Part model, mm, in its own coordinate system. A direction names the side the tool comes from. Coordinates: 2 decimals unless noted, no trailing zeros. Write each loop counter-clockwise with the first axis right and the second up, starting at its lowest first coordinate (ties: lowest second). Pieces come first, ordered by that corner, then holes. Notation, with made-up numbers: (49, 64) - (63, 64) arc R26 ccw to (63, 90) - close; hole circle Ø9 at (43, 56). An arc over 180 degrees is marked (long way). Use a Markdown table: item, result.
Autodesk Inventor part; units mm, degrees
ref_plane "Work Plane2" through (-20, 0, -10) normal (0, 0, 1) x (1, 0, 0)
ref_plane "Work Plane3" through (0, 8, 0) normal (0, 1, 0) x (1, 0, 0)
ref_plane "YZ Plane" through (0, 0, 0) normal (1, 0, 0) x (0, 1, 0)
sketch "Sketch1" plane through (0, 0, 0) normal (0, 1, 0) x (-1, 0, 0)
  line L0 (0, 0) -> (20, 0)
  line L1 (20, 0) -> (20, -20)
  line L2 (20, -20) -> (0, -20)
  line L3 (0, -20) -> (0, 0)
  dimension "d0" = 20
  dimension "d1" = 20
extrude "Extrusion1" add sketch "Sketch1" along normal blind 10
sketch "Sketch4" plane through (0, 10, 0) normal (0, 1, 0) x (1, 0, 0)
  line L0 (0, 20) -> (-20, 20)
  line L1 (-20, 20) -> (-20, 0)
  line L2 (-20, 0) -> (0, 0)
  line L3 (0, 0) -> (0, 20)
  line L4 (0, 20) -> (-20, 20)
  line L5 (-20, 20) -> (0, 0)
  line L6 (-10.1768, 10.1768) -> (-7.7019, 12.6517)
  line L7 (-7.7019, 12.6517) -> (-5.227, 10.1768)
  line L8 (-5.227, 10.1768) -> (-7.7019, 7.7019)
  line L9 (-7.7019, 7.7019) -> (-10.1768, 10.1768)
  line L10 (-10.1768, 10.1768) -> (-12.6517, 7.7019)
  line L11 (-12.6517, 7.7019) -> (-15.1265, 10.1768)
  line L12 (-15.1265, 10.1768) -> (-12.6517, 12.6517)
  line L13 (-12.6517, 12.6517) -> (-10.1768, 10.1768)
  line L14 (-12.6517, 12.6517) -> (-10.1768, 15.1265)
  line L15 (-10.1768, 15.1265) -> (-7.7019, 12.6517)
  line L16 (-7.7019, 12.6517) -> (-10.1768, 10.1768)
  line L17 (-10.1768, 10.1768) -> (-12.6517, 12.6517)
  line L18 (-12.6517, 7.7019) -> (-10.1768, 10.1768)
  line L19 (-10.1768, 10.1768) -> (-7.7019, 7.7019)
  line L20 (-7.7019, 7.7019) -> (-10.1768, 5.227)
  line L21 (-10.1768, 5.227) -> (-12.6517, 7.7019)
  dimension "d10" = 3.5
  dimension "d11" = 3.5
  dimension "d12" = 3.5
  dimension "d13" = 3.5
extrude "Extrusion3" cut sketch "Sketch4" against normal blind 8 contours L14 L15 L6 L5 | L5 L10 L11 L12 | L20 L21 L10 L5 | L5 L6 L7 L8
sketch "Sketch5" plane through (0, 10, 0) normal (0, 1, 0) x (1, 0, 0)
  line L0 (-5.227, 10.1768) -> (-10.1768, 5.227)
  line L1 (-10.1768, 5.227) -> (-15.1265, 10.1768)
  line L2 (-15.1265, 10.1768) -> (-10.1768, 15.1265)
  line L3 (-10.1768, 15.1265) -> (-5.227, 10.1768)
  line L4 (0, 20) -> (-20, 20)
  line L5 (-20, 20) -> (-20, 0)
  line L6 (-20, 0) -> (0, 0)
  line L7 (0, 0) -> (0, 20)
  line L8 (-18, 18) -> (-2, 18)
  line L9 (-2, 18) -> (-2, 2)
  line L10 (-2, 2) -> (-18, 2)
  line L11 (-18, 2) -> (-18, 18)
  line L12 (-18, 2) -> (-18, 0)
  line L13 (-2, 2) -> (-2, 0)
  line L14 (-20, 0) -> (0, 0)
  line L15 (-18, 2) -> (-20, 2)
  line L16 (-20, 20) -> (-20, 0)
  line L17 (-2, 2) -> (0, 2)
  line L18 (0, 0) -> (0, 20)
  point P0 (0, 2)
  dimension "d16" = 2
extrude "Extrusion4" add sketch "Sketch5" along normal blind 27 contours L7 L17 L9 L8 L11 L15 L5 L4
ref_plane "Work Plane1" through (-10, 10, -2) normal (1, 0, 0) x (0, 0, -1)
sketch "Sketch6" plane through (-10, 10, -2) normal (1, 0, 0) x (0, 0, -1)
  line L0 (3.227, 0) -> (8.1768, 0)
  line L1 (3.227, 0) -> (3.227, -8)
  line L2 (3.227, -8) -> (8.1768, -8)
  line L3 (8.1768, 0) -> (8.1768, -8)
  line L4 (8.1768, 0) -> (13.1265, 0)
  line L5 (8.1768, 0) -> (8.1768, -8)
  line L6 (8.1768, -8) -> (13.1265, -8)
  line L7 (13.1265, 0) -> (13.1265, -8)
  line L8 (16, 0) -> (0, 0)
  line L9 (16, 0) -> (16, 27)
  line L10 (0, 27) -> (16, 27)
  line L11 (0, 0) -> (0, 27)
  line L12 (8.1768, 0) -> (8.1768, -8)
  line L13 (8.1768, -8) -> (8.1768, -7.25)
  circle A0 centre (8.1768, -7.25) radius 0.75
  point P0 (-2, -10)
  dimension "d20" = 0.75
  dimension "d21" = 1.5
extrude "Extrusion5" cut sketch "Sketch6" along normal mid plane 27 contours A0 L3 | L3 A0
ref_plane "Work Plane2" through (-20, 0, -10) normal (0, 0, 1) x (1, 0, 0)
sketch "Sketch7" plane through (-20, 0, -10) normal (0, 0, 1) x (1, 0, 0)
  line L0 (20, 0) -> (0, 0)
  line L1 (0, 0) -> (0, 37)
  line L2 (20, 37) -> (0, 37)
  line L3 (20, 0) -> (20, 37)
  arc A0 (14.773, 3.5) -> (14.773, 2) centre (14.773, 2.75) ccw
  arc A1 (14.773, 3.5) -> (14.773, 2) centre (14.773, 2.75) ccw
  line L4 (20, 3.5) -> (20, 2)
  line L5 (20, 3.5) -> (27.5, 3.5)
  line L6 (27.5, 3.5) -> (27.5, 2)
  line L7 (27.5, 2) -> (20, 2)
  line L8 (20, 2) -> (20, 3.5)
  line L9 (20, 3.5) -> (20, 4.5)
  line L10 (20, 0) -> (20, 37)
  line L11 (27.5, 3.5) -> (27.5, 3.5246)
  line L12 (26.775, 4.2742) -> (20, 4.5)
  arc A2 (27.5, 3.5246) -> (26.775, 4.2742) centre (26.75, 3.5246) ccw
  line L13 (20, 3.5) -> (20, 2)
  line L14 (20, 2.75) -> (27.5, 2.75)
  point P0 (27.5, 4.25)
  dimension "d25" = 7.5
  dimension "d26" = 1
  dimension "d27" = 0.75
  dimension "d28" = 0.75
revolve "Revolution1" add sketch "Sketch7" angle 360 about axis through (0, 2.75, -10) along (1, 0, 0) contours L3 L12 A2 L11 L5
mirror "Mirror1" about plane through (-10, 10, -2) normal (1, 0, 0) of "Revolution1"
sketch "Sketch8" plane through (-20, 10, -2) normal (0, 0, 1) x (1, 0, 0)
  line L0 (2, 0) -> (0, 0)
  line L1 (2, 0) -> (2, 27)
  line L2 (0, 27) -> (2, 27)
  line L3 (0, 0) -> (0, 27)
  line L4 (20, 0) -> (18, 0)
  line L5 (20, 0) -> (20, 27)
  line L6 (18, 27) -> (20, 27)
  line L7 (18, 0) -> (18, 27)
  line L8 (20, 27) -> (0, 27)
  line L9 (0, 27) -> (20, 27)
  line L10 (20, 27) -> (20, 25)
  line L11 (20, 25) -> (0, 25)
  line L12 (0, 25) -> (0, 27)
  point P0 (20, -10)
  point P1 (0, 25)
  dimension "d30" = 20
  dimension "d31" = 2
extrude "Extrusion6" add sketch "Sketch8" along normal blind 2 contours L11 L3 L2 L1 | L1 L8 L7 L11 | L7 L6 L5 L11
ref_plane "Work Plane3" through (0, 8, 0) normal (0, 1, 0) x (1, 0, 0)
sketch "Sketch9" plane through (0, 8, 0) normal (0, 1, 0) x (1, 0, 0)
  line L0 (-10.1768, 15.1265) -> (-5.227, 10.1768)
  line L1 (-15.1265, 10.1768) -> (-10.1768, 15.1265)
  line L2 (-10.1768, 5.227) -> (-15.1265, 10.1768)
  line L3 (-5.227, 10.1768) -> (-10.1768, 5.227)
  line L4 (-6.6412, 10.1768) -> (-10.1768, 13.7123)
  line L5 (-10.1768, 13.7123) -> (-13.7123, 10.1768)
  line L6 (-13.7123, 10.1768) -> (-10.1768, 6.6412)
  line L7 (-10.1768, 6.6412) -> (-6.6412, 10.1768)
  point P0 (0, 0)
  dimension "d35" = 1
extrude "Extrusion7" add sketch "Sketch9" against normal blind 6
extrude "Extrusion8" cut sketch "Sketch6" along normal mid plane 27 contours A0 L3 | L3 A0
sketch "Sketch10" plane through (0, 0, 0) normal (1, 0, 0) x (0, 0, -1)
  line L0 (0, 0) -> (20, 0)
  line L1 (20, 0) -> (20, 37)
  line L2 (20, 37) -> (0, 37)
  line L3 (0, 35) -> (0, 37)
  line L4 (2, 35) -> (0, 35)
  line L5 (2, 10) -> (2, 35)
  line L6 (0, 10) -> (2, 10)
  line L7 (0, 0) -> (0, 10)
  circle A0 centre (10, 2.75) radius 1.75
  line L8 (2, 35) -> (10, 35)
  line L9 (10, 35) -> (4.5, 35)
  line L10 (4.5, 35) -> (4.5, 30)
  line L11 (4.5, 30) -> (17, 30)
  line L12 (17, 30) -> (17, 17.5)
  line L13 (17, 17.5) -> (4.5, 17.5)
  line L14 (4.5, 17.5) -> (4.5, 30)
  dimension "d40" = 5.5
  dimension "d41" = 5
  dimension "d42" = 12.5
  dimension "d43" = 12.5
  dimension "d44" = 8
extrude "Extrusion9" cut sketch "Sketch10" against normal blind 6 contours L11 L12 L13 L14
properties part number "latticeChamberv4"
Item 1: Band-saw the part on A-A, the plane y = 24.5. Give the cut face in (x, z), then the cut area to 3 significant figures.
From the geometry:
| item | result |
|---|---|
| outline | (-20, -20) - (0, -20) - (0, -17) - (-2, -17) - (-2, -18) - (-18, -18) - (-18, -2) - (-20, -2) - close; (-2, -4.5) - (0, -4.5) - (0, -2) - (-2, -2) - close |
| area | 79.0 mm^2 |
Item 2: Band-saw the part on C-C, the plane x = -19.5. Give the cut face in (y, z).
From the geometry:
| item | result |
|---|---|
| outline | (0, -20) - (37, -20) - (37, 0) - (35, 0) - (35, -2) - (10, -2) - (10, 0) - (0, 0) - close; hole circle Ø1.5 at (2.75, -10.18) |
Item 3: Band-saw the part on D-D, the plane z = -14.5. Give the cut face in (x, y).
From the geometry:
| item | result |
|---|---|
| outline | (-20, 0) - (0, 0) - (0, 17.5) - (-2, 17.5) - (-2, 10) - (-9.55, 10) - (-9.55, 8) - (-10.8, 8) - (-10.8, 10) - (-18, 10) - (-18, 37) - (-20, 37) - close; (-2, 30) - (0, 30) - (0, 37) - (-2, 37) - close |
Item 4: Drill centre lines: probe 1 along Y at (x, z) = (-1.5, -5.5); probe 2 along X at (y, z) = (10.5, -14.5); probe 3 along Z at (x, y) = (-17.5, 10.5). Where is each one in solid material? Low to high.
From the geometry:
| item | result |
|---|---|
| probe 1 | 0 to 17.5, 30 to 37 |
| probe 2 | -20 to -18, -2 to 0 |
| probe 3 | -20 to -18 |
Item 5: Band-saw the part on B-B, the plane y = 7.5. Give the cut face in (x, z).
From the geometry:
| item | result |
|---|---|
| outline | (-20, -20) - (0, -20) - (0, 0) - (-20, 0) - close; hole (-13.71, -10.18) - (-10.18, -13.71) - (-6.64, -10.18) - (-10.18, -6.64) - close |
Item 6: Drop flat-ended pins along their axis: P1, Ø0.9, axis at y = 2.75, z = -10, coming from the +X side; P2, Ø3, axis at x = -15.5, z = -15.5, coming from the -Y side; P3, Ø1, axis at y = 32.5, z = -16.5, coming from the -X side; P4, Ø0.6, axis at x = -1, y = 28.5, coming from the +Z side. Give the stop position or say it passes through.
From the geometry:
| item | result |
|---|---|
| P1 | through |
| P2 | y = 0 |
| P3 | x = -20 |
| P4 | z = -2 |
Item 7: Which spindle directions (+Z, -Z, +X, -X, +Y, -Y) get a long thin tool onto all of the face, cutting with end or side? Do faces 1 (the face through (-1, 24, -4.5)), 2 (the face through (-16.98, 2.98, -10.89)), 3 (the face through (-8.434, 5.042, -8.384)). Say none if no direction does.
From the geometry:
| item | result |
|---|---|
| face 1 | +X |
| face 2 | none |
| face 3 | +Y |
Item 8: Two-plate mould, pull along X, no slides. Class faces 4 (the face through (-8, 10, -7)), 5 (the face through (-1, 22, -2)), 6 (the face through (-20, 18, -10)), 7 (the face through (-3.08, 2.98, -10.89)): pulls with the +X half, pulls with the -X half, needs draft (parallel to the pull), parting line crosses it, or undercut.
From the geometry:
| item | result |
|---|---|
| face 4 | undercut |
| face 5 | needs draft |
| face 6 | pulls with the -X half |
| face 7 | undercut |
